Source: CAD feature listing. Evaluate the final solid. Frame: model axes, mm. A direction names the side the tool comes from. Give positions to 0.01 mm unless a question says otherwise; leave off trailing zeros. Order: outer loops, then holes, each group sorted by start corner. A loop starts at its lowest first (then second) coordinate and runs counter-clockwise, first axis right, second up. Notation, with made-up numbers: M 87,1.25 L 107,1.25 A22 cw 107,39.25 Z; hole C 58.5,-23.75 d1. An arc over 180 degrees is marked long. Return JSON: item names as keys, results as strings.
from build123d import *

# Parameters (mm, degrees)
F0_W      = 80
F0_H      = 12
F1_DEPTH  = 10
F2_R      = 5.05
F3_DEPTH  = 4
F4_R      = 5
F5_R      = 5
F6_R      = 1.75
F7_DEPTH  = 25
F8_R      = 0.5
F9_R      = 0.5
F10_R     = 1.75
F11_DEPTH = 25
F12_R     = 1
F13_DEPTH = 25


with BuildPart() as f1:
    # F0 (on Top) → F1 (new body)
    with BuildSketch(Plane.XY):
        Rectangle(F0_W, F0_H)
    extrude(amount=F1_DEPTH)

    # F2 (on face) → F3 (cut)
    with BuildSketch(Plane.XY.offset(10)):
        with Locations((34, 0)):
            Circle(F2_R)
        with Locations((23, 0)):
            Circle(F2_R)
        with Locations((12, 0)):
            Circle(F2_R)
        with Locations((1, 0)):
            Circle(F2_R)
        with Locations((-10, 0)):
            Circle(F2_R)
        with Locations((-21, 0)):
            Circle(F2_R)
    extrude(amount=-F3_DEPTH, mode=Mode.SUBTRACT)

    # F4
    f4_edges = [f1.edges().sort_by_distance(p)[0] for p in [
        (40, -6, 5),
    ]]
    fillet(f4_edges, radius=F4_R)

    # F5
    f5_edges = [f1.edges().sort_by_distance(p)[0] for p in [
        (40, 6, 5),
        (-40, -6, 5),
        (-40, 6, 5),
    ]]
    fillet(f5_edges, radius=F5_R)

    # F6 (on face) → F7 (cut)
    with BuildSketch(Plane.XY.offset(6)):
        with Locations((34, 0)):
            Circle(F6_R)
        with Locations((23, 0)):
            Circle(F6_R)
        with Locations((12, 0)):
            Circle(F6_R)
        with Locations((1, 0)):
            Circle(F6_R)
        with Locations((-10, 0)):
            Circle(F6_R)
        with Locations((-21, 0)):
            Circle(F6_R)
    extrude(amount=-F7_DEPTH, mode=Mode.SUBTRACT)

    # F8
    f8_edges = [f1.edges().sort_by_distance(p)[0] for p in [
        (0, -6, 10),
        (38.535534, -4.535534, 10),
        (38.535534, 4.535534, 10),
        (0, 6, 10),
        (-38.535534, -4.535534, 10),
    ]]
    fillet(f8_edges, radius=F8_R)

    # F9
    f9_edges = [f1.edges().sort_by_distance(p)[0] for p in [
        (0, -6, 0),
        (-38.535534, -4.535534, 0),
        (0, 6, 0),
        (38.535534, 4.535534, 0),
        (38.535534, -4.535534, 0),
    ]]
    fillet(f9_edges, radius=F9_R)

    # F10 (on face) → F11 (cut)
    with BuildSketch(Plane(origin=(0, 0, 0), x_dir=(1, 0, 0), z_dir=(0, 0, -1))):
        with Locations((-34, 0.0696202532)):
            Circle(F10_R)
    extrude(amount=-F11_DEPTH, mode=Mode.SUBTRACT)

    # F12 (on face) → F13 (cut)
    with BuildSketch(Plane(origin=(0, 6, 0), x_dir=(-1, 0, 0), z_dir=(0, 1, 0))):
        with Locations((34, 5)):
            Circle(F12_R)
    extrude(amount=-F13_DEPTH, mode=Mode.SUBTRACT)


solid = f1.part
1. Ray query, probe 1 along Y at (x, z) = (-10, 9.25); probe 2 along Z at (x, y) = (-18.5, 1.75); probe 3 along X at (y, z) = (3.45, 5). Return the intervals inside material, ascending.
Evaluation:
{"probe 1": "y = -6 to -5.05, 5.05 to 6", "probe 2": "z = 0 to 6", "probe 3": "x = -39.36 to -35, -33 to 39.36"}
2. Draft query along X for faces 1 (the face through (-0.75, 0.08, 3.04)), 2 (the face through (-38, -5, 5)), 3 (the face through (32.71, 1.18, 3.04)), 4 (the face through (40, 0, 5)). Return one class per face: pulls with the +X half, pulls with the -X half, needs draft (parallel to the pull), parting line crosses it, or undercut.
Evaluation:
{"face 1": "undercut", "face 2": "pulls with the -X half", "face 3": "undercut", "face 4": "pulls with the +X half"}
3. Set-up query: faces 5 (the face through (13.669, 0.526, 3.042)), 6 (the face through (36, 0, 6)). Return all of +Z, -Z, +X, -X, +Y, -Y with unobstructed straight access to the full face (end or side cutting, diameter ignored); none if empty.
Evaluation:
{"face 5": "+Z, -Z", "face 6": "+Z"}
4. Section query A-A (x = 34). Return loops of the section in (y, z).
Evaluation:
{"outline": "M -6,0.5 A0.5 ccw -5.5,0 L -1.75,0 L -1.75,6 L -5.05,6 L -5.05,10 L -5.5,10 A0.5 ccw -6,9.5 Z; M 1.75,0 L 5.5,0 A0.5 ccw 6,0.5 L 6,9.5 A0.5 ccw 5.5,10 L 5.05,10 L 5.05,6 L 1.75,6 Z"}
5. First-contact query: pin 1 (6 mm diameter, centred on x = 19, y = -1, fed in from +Z); pin 2 (5 mm diameter, centred on x = 32.5, y = -1, fed in from +Z). Flat tips, straight axial feed; report the tip coordinate or a pass-through.
Evaluation:
{"pin 1": "stops at z = 10", "pin 2": "stops at z = 6"}
6. Section query B-B (z = 1.5). Return loops of the section in (x, y).
Evaluation:
{"outline": "M -40,-1 A5 ccw -35,-6 L 35,-6 A5 ccw 40,-1 L 40,1 A5 ccw 35,6 L -35,6 A5 ccw -40,1 Z; hole C -34,-0.07 d3.5; hole C -21,0 d3.5; hole C -10,0 d3.5; hole C 1,0 d3.5; hole C 12,0 d3.5; hole C 23,0 d3.5; hole C 34,0 d3.5"}
